Check sheet for the drawn part. Datum: minimum x, y, z corner. Units: mm. Coordinates: 2 decimals unless noted, no trailing zeros. Loops run counter-clockwise (first coordinate to the right, second up) from the corner with the lowest first, then second, coordinate; pieces in that order, holes last.
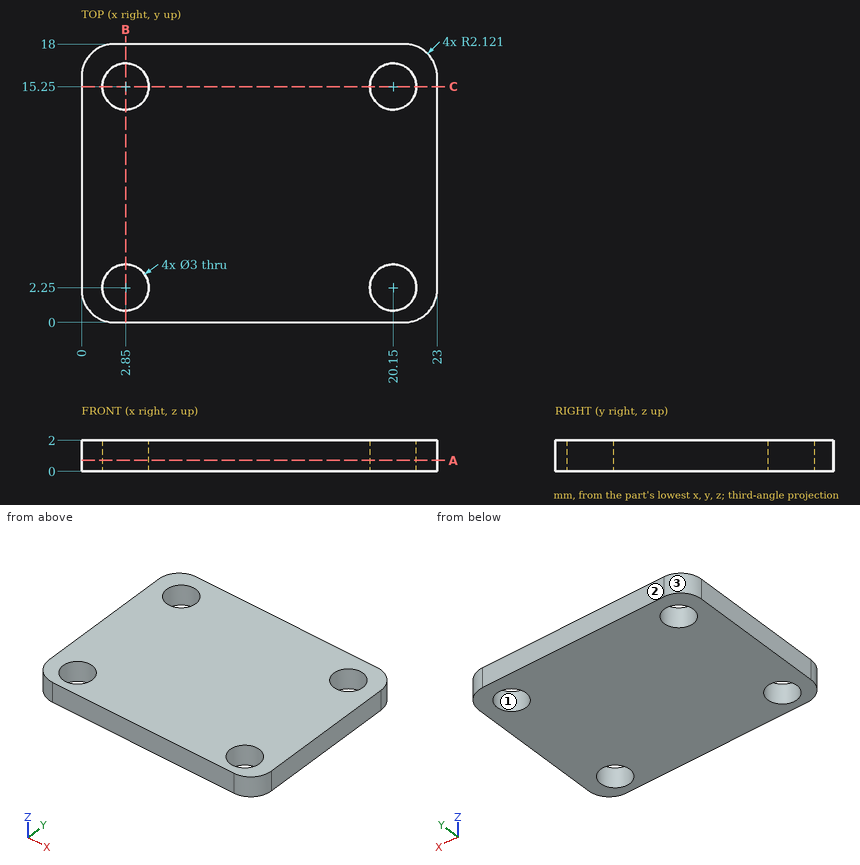
1) Section check B-B on x = 2.85. Enter the section's corners in (y, z), plus the area to 3 significant figures.
Answer sheet:
outline: (0, 0) - (0.75, 0) - (0.75, 2) - (0, 2) - close; (3.75, 0) - (13.75, 0) - (13.75, 2) - (3.75, 2) - close; (16.75, 0) - (18, 0) - (18, 2) - (16.75, 2) - close
area: 24.0 mm2
2) Section check C-C on y = 15.25. Enter the section's corners in (x, z), plus the area to 3 significant figures.
Answer sheet:
outline: (0, 0) - (1.35, 0) - (1.35, 2) - (0, 2) - close; (4.35, 0) - (18.65, 0) - (18.65, 2) - (4.35, 2) - close; (21.65, 0) - (23, 0) - (23, 2) - (21.65, 2) - close
area: 34.0 mm2
3) Scan lines: line 1 (Y direction, x = 20.15, z = 0.85); line 2 (Y direction, x = 19.5, z = 1.85); line 3 (X direction, y = 1.25, z = 1.25). Record each from-to range of solid material in increasing order.
Answer sheet:
line 1: y = 0 to 0.75, 3.75 to 13.75, 16.75 to 18
line 2: y = 0 to 0.9, 3.6 to 13.9, 16.6 to 18
line 3: x = 0.19 to 1.73, 3.97 to 19.03, 21.27 to 22.81
4) Depth check by flat-ended pin: pin 1 (1 mm diameter, centred on x = 3, y = 5.5, fed in from -Z); pin 2 (2.5 mm diameter, centred on x = 20.15, y = 2.25, fed in from -Z). Enter the tip coordinate at first touch or a pass-through.
Answer sheet:
pin 1: stops at z = 0
pin 2: passes through
5) Section check A-A on z = 0.7. Enter the section's corners in (x, y), plus the area to 3 significant figures.
Answer sheet:
outline: (0, 2.12) arc R2.12 ccw to (2.12, 0) - (20.88, 0) arc R2.12 ccw to (23, 2.12) - (23, 15.88) arc R2.12 ccw to (20.88, 18) - (2.12, 18) arc R2.12 ccw to (0, 15.88) - close; hole circle Ø3 at (2.85, 2.25); hole circle Ø3 at (2.85, 15.25); hole circle Ø3 at (20.15, 2.25); hole circle Ø3 at (20.15, 15.25)
area: 382 mm2
6) Mould release check, pull along X, two halves, no side actions. Record for the marked faces 1, 2 and 3: +X half, -X half, draft (parallel to the pull), parting line (faces both ways), or undercut.
Answer sheet:
face 1: undercut
face 2: draft
face 3: -X half
